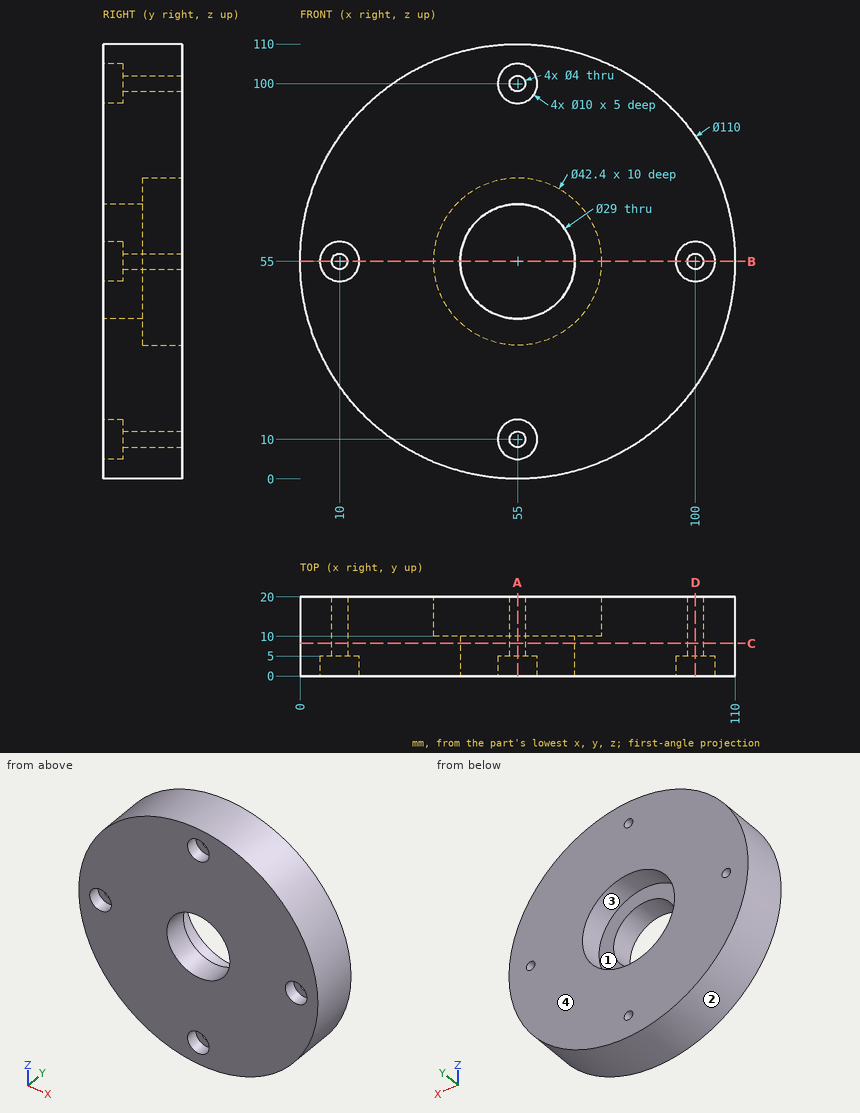
The figure shows three views and two pictorial views of one solid part (mm, origin at its lowest corner). Answer the questions. Give positions to 0.01 mm unless a question says otherwise; leave off trailing zeros. Order: outer loops, then holes, each group sorted by start corner. A loop starts at its lowest first (then second) coordinate and runs counter-clockwise, first axis right, second up. Notation, with made-up numbers: (16, 40) -> (37, 40) arc R14 ccw to (37, 44) -> close; hole circle Ø11 at (79.25, -20). An arc over 180 degrees is marked (long way). Write each question's results on one line, items separated by ' | '.
Q1. The part is cut by section D-D, the plane x = 100. Give the vertices of the cut face in (y, z).
Checked values:
outline: (0, 23.38) -> (20, 23.38) -> (20, 53) -> (5, 53) -> (5, 50) -> (0, 50) -> close; (0, 60) -> (5, 60) -> (5, 57) -> (20, 57) -> (20, 86.62) -> (0, 86.62) -> close
Q2. Each of these flat-tipped pins is pushed along its axis until it touches: P1, Ø8, axis at x = 55, z = 100, coming from the -Y side; P2, Ø1, axis at y = 12.5, z = 64, coming from the -X side. Where does it stop, or does it pass through?
Checked values:
P1: stops at y = 5 | P2: stops at x = 0.66
Q3. The part is cut by section C-C, the plane y = 8.25. Give the vertices of the cut face in (x, z), and give its area (3 significant figures).
Checked values:
outline: circle Ø110 at (55, 55); hole circle Ø4 at (10, 55); hole circle Ø29 at (55, 55); hole circle Ø4 at (55, 10); hole circle Ø4 at (55, 100); hole circle Ø4 at (100, 55) | area: 8,790 mm^2
Q4. The part is cut by section A-A, the plane x = 55. Give the vertices of the cut face in (y, z), and give its area (3 significant figures).
Checked values:
outline: (0, 0) -> (20, 0) -> (20, 8) -> (5, 8) -> (5, 5) -> (0, 5) -> close; (0, 15) -> (5, 15) -> (5, 12) -> (20, 12) -> (20, 33.8) -> (10, 33.8) -> (10, 40.5) -> (0, 40.5) -> close; (0, 69.5) -> (10, 69.5) -> (10, 76.2) -> (20, 76.2) -> (20, 98) -> (5, 98) -> (5, 95) -> (0, 95) -> close; (0, 105) -> (5, 105) -> (5, 102) -> (20, 102) -> (20, 110) -> (0, 110) -> close | area: 1,270 mm^2
Q5. Straight lines are drawn through the part: probe 1 along X at (y, z) = (6, 55); probe 2 along Z at (x, y) = (55, 1.1); probe 3 along Y at (x, z) = (43, 67.5). For each, find the intervals that lie inside material, in ascending order. Write a range as from..to.
Checked values:
probe 1: x = 0..8, 12..40.5, 69.5..98, 102..110 | probe 2: z = 0..5, 15..40.5, 69.5..95, 105..110 | probe 3: y = 0..10
Q6. Determine the mould class of the marked faces 1, 2, 3 and 4 for opening direction X: pulls with the +X half, pulls with the -X half, needs draft (parallel to the pull), parting line crosses it, or undercut.
Checked values:
face 1: undercut | face 2: parting line crosses it | face 3: undercut | face 4: needs draft
Q7. The part is cut by section B-B, the plane z = 55. Give the vertices of the cut face in (x, y).
Checked values:
outline: (0, 0) -> (5, 0) -> (5, 5) -> (8, 5) -> (8, 20) -> (0, 20) -> close; (12, 5) -> (15, 5) -> (15, 0) -> (40.5, 0) -> (40.5, 10) -> (33.8, 10) -> (33.8, 20) -> (12, 20) -> close; (69.5, 0) -> (95, 0) -> (95, 5) -> (98, 5) -> (98, 20) -> (76.2, 20) -> (76.2, 10) -> (69.5, 10) -> close; (102, 5) -> (105, 5) -> (105, 0) -> (110, 0) -> (110, 20) -> (102, 20) -> close
